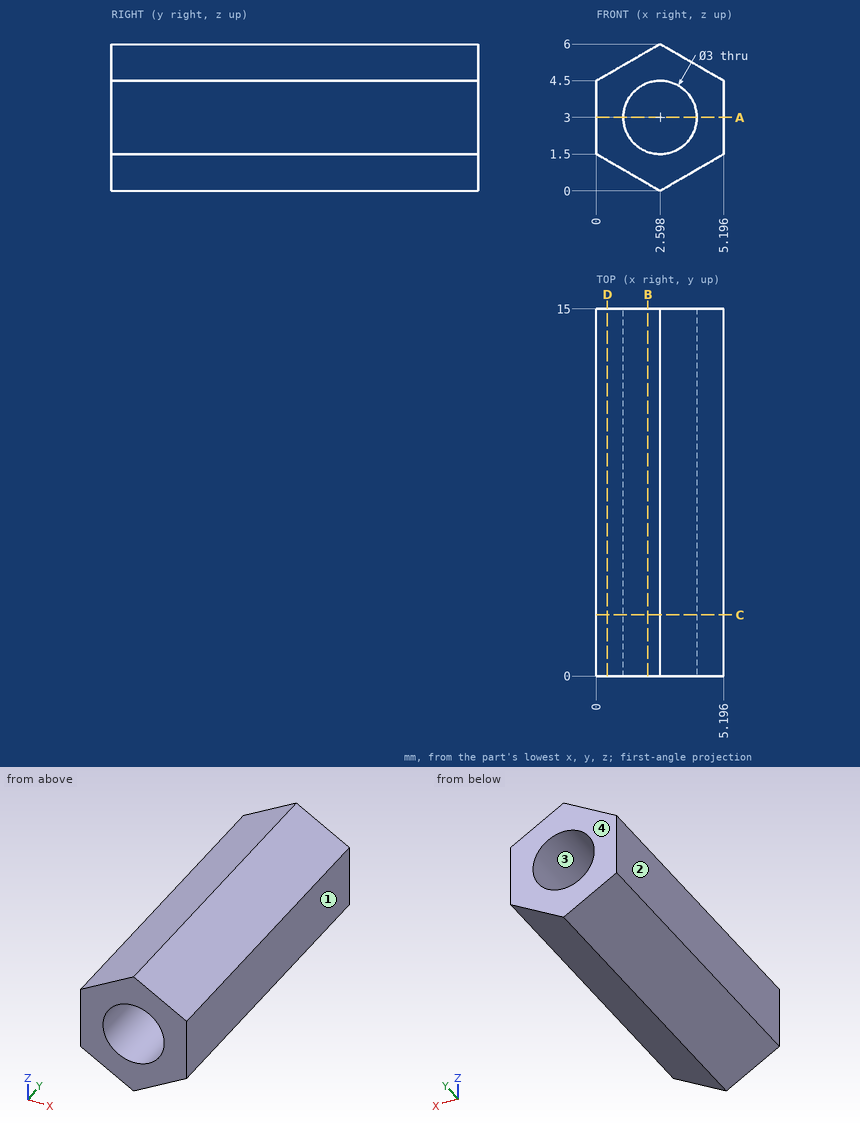
Design review of the part shown in the three views and the two pictorial views. Dimensions are in mm from the part's minimum x, y and z. Coordinates: 2 decimals unless noted, no trailing zeros. Loops run counter-clockwise (first coordinate to the right, second up) from the corner with the lowest first, then second, coordinate; pieces in that order, holes last. Notation, with made-up numbers: M 81.25,-5 L 110.25,-5 A22 ccw 110.25,7 Z; hole C 59.25,79.5 d9. An arc over 180 degrees is marked long. Put each result on its own line as item: value. Start each with the question number.
Q1. The part is to be moulded in two halves that separate along X. For the marked faces 1, 2, 3 and 4, say which applies: +X half, -X half, draft (parallel to the pull), parting line (faces both ways), or undercut.
Q2. Add section C-C (y = 2.5). Write out the cut boundary in (x, z).
Q3. Add section D-D (x = 0.45). Write out the cut boundary in (y, z), and give its area (3 significant figures).
Q4. Add section B-B (x = 2.1). Write out the cut boundary in (y, z) (1 decimal).
Q5. Add section A-A (z = 3). Write out the cut boundary in (x, y).
Q6. Wall thickness on line 1 (X direction, y = 12.25, z = 3); line 2 (Z direction, x = 1.4, y = 1); line 3 (Z direction, x = 3.6, y = 12): over which ranges is each line inside the solid? List them lowest first.
Q7. Clearance check with flat-ended pins moving along their axes: pin 1 (2 mm diameter, centred on x = 1.5, y = 7.5, fed in from +Z); pin 2 (3 mm diameter, centred on x = 4.5, y = 12.5, fed in from -Z). State where each tip first meets the part, or that it passes through.
Answers:
1. face 1: +X half
1. face 2: -X half
1. face 3: undercut
1. face 4: draft
2. outline: M 0,1.5 L 2.6,0 L 5.2,1.5 L 5.2,4.5 L 2.6,6 L 0,4.5 Z; hole C 2.6,3 d3
3. outline: M 0,1.24 L 15,1.24 L 15,4.76 L 0,4.76 Z
3. area: 52.8 mm^2
4. outline: M 0,0.3 L 15,0.3 L 15,1.6 L 0,1.6 Z; M 0,4.4 L 15,4.4 L 15,5.7 L 0,5.7 Z
5. outline: M 0,0 L 1.1,0 L 1.1,15 L 0,15 Z; M 4.1,0 L 5.2,0 L 5.2,15 L 4.1,15 Z
6. line 1: x = 0 to 1.1, 4.1 to 5.2
6. line 2: z = 0.69 to 2.1, 3.9 to 5.31
6. line 3: z = 0.58 to 1.88, 4.12 to 5.42
7. pin 1: stops at z = 5.94
7. pin 2: stops at z = 0.23
